Here's the drawing with two shaded views (mm, measured from the low corner). I have some questions. Round coordinates to 2 decimals unless told otherwise and drop trailing zeros. Loops run counter-clockwise (first coordinate to the right, second up) from the corner with the lowest first, then second, coordinate; pieces in that order, holes last.
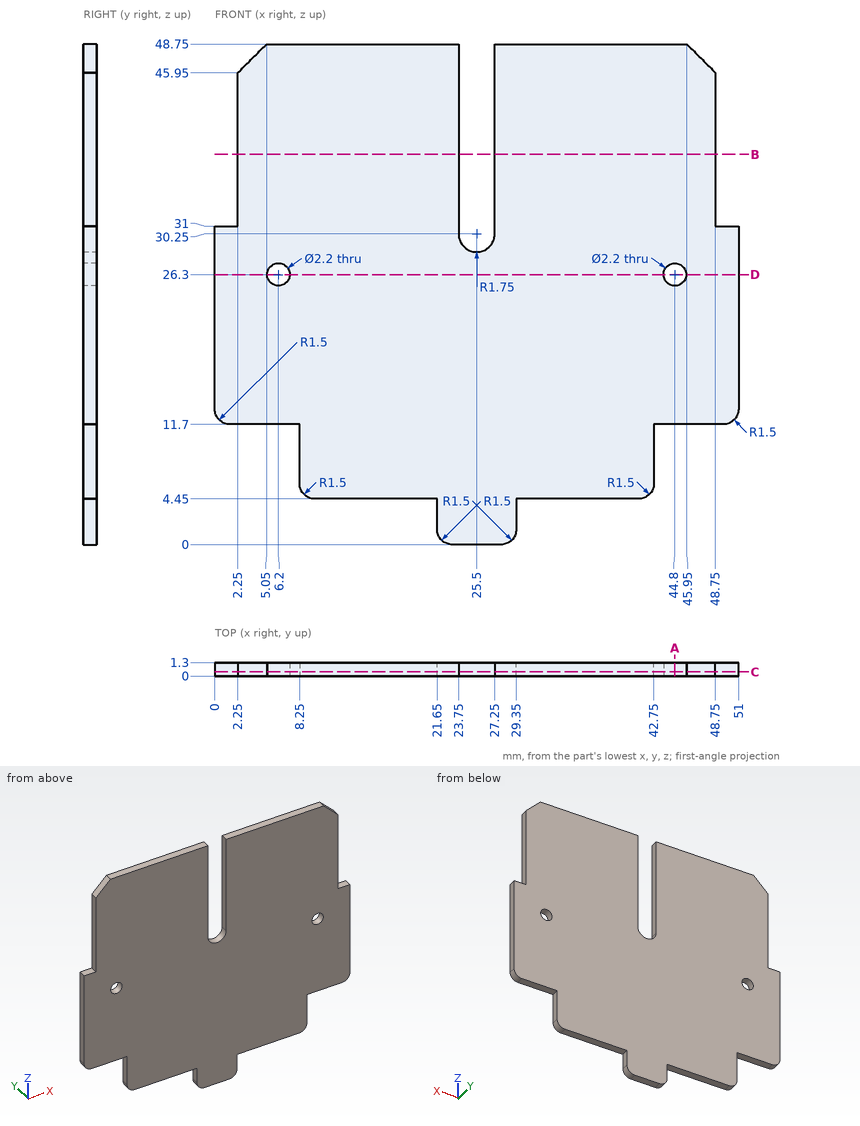
Item 1: If I drill on line 1 along X through (y, z) = (0.7, 26.3); line 2 along X through (y, z) = (0.25, 36.5); line 3 along Z through (x, y) = (16.5, 0.65), over which ranges is the centre line in solid material (lowest first)?
Results list:
line 1: x = 0 to 5.1, 7.3 to 43.7, 45.9 to 51
line 2: x = 2.25 to 23.75, 27.25 to 48.75
line 3: z = 4.45 to 48.75
Item 2: If we section it at D-D, the plane z = 26.3: Please give me the cut outline in (x, y).
Results list:
outline: (0, 0) - (5.1, 0) - (5.1, 1.3) - (0, 1.3) - close; (7.3, 0) - (43.7, 0) - (43.7, 1.3) - (7.3, 1.3) - close; (45.9, 0) - (51, 0) - (51, 1.3) - (45.9, 1.3) - close
Item 3: Will these pins go through, and if not, where does the flat tip stop? pin 1 (2 mm diameter, centred on x = 13, z = 41.5, fed in from -Y); pin 2 (0.6 mm diameter, centred on x = 44.5, y = 0.5, fed in from -Z).
Results list:
pin 1: stops at y = 0
pin 2: stops at z = 11.7
Item 4: If we section it at C-C, the plane y = 0.4: Count the separate pieces of the cut face and the enclosed holes in it, then the cut area to 3 significant figures.
Results list:
separate pieces: 1
enclosed holes: 2
area: 2,010 mm2
Item 5: If we section it at B-B, the plane z = 38: Please give me the cut outline in (x, y), then the cut area to 3 significant figures.
Results list:
outline: (2.25, 0) - (23.75, 0) - (23.75, 1.3) - (2.25, 1.3) - close; (27.25, 0) - (48.75, 0) - (48.75, 1.3) - (27.25, 1.3) - close
area: 55.9 mm2
Item 6: If we section it at A-A, the plane x = 44.8: Please give me the cut outline in (y, z).
Results list:
outline: (0, 11.7) - (1.3, 11.7) - (1.3, 25.2) - (0, 25.2) - close; (0, 27.4) - (1.3, 27.4) - (1.3, 48.75) - (0, 48.75) - close
